Here's how the part is built. I have some questions about the finished solid (model axes, mm). A direction names the side the tool comes from. Round coordinates to 2 decimals unless told otherwise and drop trailing zeros. Write each loop counter-clockwise with the first axis right and the second up, starting at its lowest first coordinate (ties: lowest second). Pieces come first, ordered by that corner, then holes. Notation, with made-up numbers: (36.5, 84.25) -> (63.5, 84.25) arc R37 ccw to (63.5, 121.25) -> close; hole circle Ø6 at (33, 67.5). An arc over 180 degrees is marked (long way). Answer in a Markdown table with one row per item.
Autodesk Inventor part; units mm, degrees
ref_plane "YZ Plane" through (0, 0, 0) normal (1, 0, 0) x (0, 1, 0)
ref_plane "XZ Plane" through (0, 0, 0) normal (0, 1, 0) x (-1, 0, 0)
ref_plane "XY Plane" through (0, 0, 0) normal (0, 0, 1) x (1, 0, 0)
sketch "Sketch1" plane through (0, 0, 0) normal (0, 0, 1) x (1, 0, 0)
  line L0 (0, 64) -> (0, 0)
  line L1 (24.8907, 0) -> (21.3073, 0)
  line L2 (0, 64) -> (8, 64)
  line L3 (33.8546, 8) -> (33.8546, 0)
  line L4 (33.8546, 0) -> (0, 0)
  line L5 (0, 0) -> (0, 64)
  line L6 (8, 64) -> (8, 8)
  line L7 (8, 8) -> (33.8546, 8)
  line L8 (33.8546, 8) -> (8, 33.8546)
  line L9 (33.8546, 8) -> (70.4186, 8) construction
  point P0 (0, 0)
  dimension "d0" = 8
  dimension "d1" = 8
  dimension "d2" = 135
  dimension "d9" = 64
extrude "Extrusion1" add sketch "Sketch1" along normal blind 3
extrude "Extrusion2" add sketch "Sketch1" against normal blind 10 contours L2 L6 L7 L3 L4 L1 L0
extrude "Extrusion3" add sketch "Sketch1" against normal blind 3 from surface at -10
sketch "Sketch2" plane through (8, 33.8546, 3) normal (1, 0, 0) x (0, 0, -1)
  circle A0 centre (8, 11.1454) radius 2.5
  circle A1 centre (8, -20.8546) radius 2.5
  line L0 (16, 30.1454) -> (0, 30.1454)
  line L1 (8, 30.1454) -> (8, -25.8546) construction
  line L2 (3, -25.8546) -> (13, -25.8546) construction
  point P0 (3, -33.8546)
  dimension "d20" = 32
  dimension "d21" = 19
extrude "Extrusion4" cut sketch "Sketch2" against normal through all
sketch "Sketch3" plane through (8, 8, 0) normal (0, 1, 0) x (1, 0, 0)
  circle A0 centre (15.0917, 5) radius 2.8
  line L0 (0, 0) -> (0, 10)
  line L1 (0, 7.5) -> (0, 2.5) construction
  line L2 (0, 5) -> (22.225, 5) construction
  line L3 (0, 5) -> (22.225, 5) construction
  line L4 (10.9735, 7.4504) -> (15.1547, 9.7916)
  line L5 (15.1547, 9.7916) -> (19.2728, 7.3412)
  line L6 (19.2728, 7.3412) -> (19.2098, 2.5496)
  line L7 (19.2098, 2.5496) -> (15.0287, 0.2084)
  line L8 (15.0287, 0.2084) -> (10.9105, 2.6588)
  line L9 (10.9105, 2.6588) -> (10.9735, 7.4504)
  point P0 (-8, 0)
  dimension "d13" = 5.6
  dimension "d14" = 0
  dimension "d22" = 8.3
extrude "Extrusion5" cut sketch "Sketch3" against normal through all contours A0
extrude "Extrusion7" cut sketch "Sketch3" against normal blind 4 contours A0 | L4 L5 L6 L7 L8 L9
equation "\"d1\" = d0"
properties part number "Lower Limit Switch"
1) I want a section at C-C, the plane z = -5. List the corners of the cut face in (x, y) for me.
Response:
| item | result |
|---|---|
| outline | (0, 0) -> (20.29, 0) -> (20.29, 4) -> (18.94, 4) -> (18.94, 8) -> (8, 8) -> (8, 10.5) -> (0, 10.5) -> close; (0, 15.5) -> (8, 15.5) -> (8, 42.5) -> (0, 42.5) -> close; (0, 47.5) -> (8, 47.5) -> (8, 64) -> (0, 64) -> close; (25.89, 0) -> (33.85, 0) -> (33.85, 8) -> (27.24, 8) -> (27.24, 4) -> (25.89, 4) -> close |
2) For pin 1 (5 mm diameter, centred on y = 36, z = -5, fed in from +X); pin 2 (12 mm diameter, centred on x = 28, y = 16.5, fed in from +Z); pin 3 (4.5 mm diameter, centred on x = 23.09, z = -5, fed in from +Y); pin 4 (4 mm diameter, centred on x = 24, z = -3.5, fed in from +Y), each with a flat end and sliding along its axis, tell me the tip position at first contact or that it passes through.
Response:
| item | result |
|---|---|
| pin 1 | stops at x = 8 |
| pin 2 | stops at z = 3 |
| pin 3 | passes through |
| pin 4 | stops at y = 4 |
3) We'd pull the mould along Y, two halves only. Please class faces 4 (the face through (9, 25, 3)), 5 (the face through (4.06, 42.56, -4.46)), 6 (the face through (4.06, 10.78, -6.15)), 7 (the face through (20, 4, -5)): +Y half, -Y half, draft (parallel to the pull), parting line (faces both ways), or undercut.
Response:
| item | result |
|---|---|
| face 4 | draft |
| face 5 | undercut |
| face 6 | undercut |
| face 7 | +Y half |
4) I want a section at B-B, the plane x = 2. List the corners of the cut face in (y, z) for me, and give its area (3 significant figures).
Response:
| item | result |
|---|---|
| outline | (0, -13) -> (64, -13) -> (64, 3) -> (0, 3) -> close; hole circle Ø5 at (13, -5); hole circle Ø5 at (45, -5) |
| area | 985 mm^2 |
5) I want a section at D-D, the plane z = 1.5. List the corners of the cut face in (x, y) for me, and give its area (3 significant figures).
Response:
| item | result |
|---|---|
| outline | (0, 0) -> (33.85, 0) -> (33.85, 8) -> (8, 33.85) -> (8, 64) -> (0, 64) -> close |
| area | 1,050 mm^2 |
6) I want a section at A-A, the plane y = 45. List the corners of the cut face in (x, z) for me.
Response:
| item | result |
|---|---|
| outline | (0, -13) -> (8, -13) -> (8, -7.5) -> (0, -7.5) -> close; (0, -2.5) -> (8, -2.5) -> (8, 3) -> (0, 3) -> close |
7) I need wall thicknesses on line 1 (Y direction, x = 4.5, z = -5); line 2 (X direction, y = 2.8, z = -5); line 3 (Z direction, x = 13, y = 12). Which ranges of each line are inside material? Lowest first, please. Write a range as [from, to].
Response:
| item | result |
|---|---|
| line 1 | y = [0, 10.5], [15.5, 42.5], [47.5, 64] |
| line 2 | x = [0, 20.29], [25.89, 33.85] |
| line 3 | z = [-13, -10], [0, 3] |
8) Which directions (+Z, -Z, +X, -X, +Y, -Y) give clear straight access to the entire face, cutting with the end or side of a thin tool? Please do faces 1 (the face through (25.149, 6.028, -1.395)), 2 (the face through (21.108, 20.746, -11.479)), 3 (the face through (18, 8, -5)).
Response:
| item | result |
|---|---|
| face 1 | +Y |
| face 2 | +Z, -Z, +X, +Y |
| face 3 | +X, +Y |
